```python
from build123d import *

# Parameters (mm, degrees)
F0_R     = 25.4
F0_R_2   = 9.525
F1_DEPTH = 6.35
F2_SIZE  = 5.08


with BuildPart() as f1:
    # F0 (on Front) → F1 (new body)
    with BuildSketch(Plane.XZ):
        with BuildLine():
            Line((109.5375, 0), (1.5875, 0))
            ThreePointArc((1.5875, 0), (1.122532, -1.122532), (0, -1.5875))
            Line((0, -1.5875), (0, -169.8625))
            ThreePointArc((0, -169.8625), (1.122532, -170.327468), (1.5875, -171.45))
            Line((1.5875, -171.45), (109.5375, -171.45))
            ThreePointArc((109.5375, -171.45), (110.002468, -170.327468), (111.125, -169.8625))
            Line((111.125, -169.8625), (111.125, -90.614297))
            ThreePointArc((111.125, -90.614297), (52.3875, -50.8), (111.125, -10.985703))
            Line((111.125, -10.985703), (111.125, -1.5875))
            ThreePointArc((111.125, -1.5875), (110.002468, -1.122532), (109.5375, 0))
        make_face()
        with Locations((77.7875, -142.875)):
            Circle(F0_R, mode=Mode.SUBTRACT)
        with Locations((38.1, -101.6)):
            Circle(F0_R, mode=Mode.SUBTRACT)
        with BuildLine():
            ThreePointArc((0, -1.5875), (-1.122532, 1.122532), (1.5875, 0))
            Line((1.5875, 0), (109.5375, 0))
            ThreePointArc((109.5375, 0), (110.002468, 1.122532), (111.125, 1.5875))
            Line((111.125, 1.5875), (111.125, 14.2875))
            Line((111.125, 14.2875), (-19.05, 14.2875))
            Line((-19.05, 14.2875), (-19.05, -185.7375))
            Line((-19.05, -185.7375), (121.44375, -185.7375))
            Line((121.44375, -185.7375), (121.44375, -129.918501))
            ThreePointArc((121.44375, -129.918501), (135.685573, -89.928697), (174.625, -73.025))
            Line((174.625, -73.025), (174.625, 0))
            Line((174.625, 0), (112.7125, 0))
            ThreePointArc((112.7125, 0), (112.247532, -1.122532), (111.125, -1.5875))
            Line((111.125, -1.5875), (111.125, -10.985703))
            ThreePointArc((111.125, -10.985703), (130.729826, -26.750554), (138.1125, -50.8))
            ThreePointArc((138.1125, -50.8), (130.729826, -74.849446), (111.125, -90.614297))
            Line((111.125, -90.614297), (111.125, -169.8625))
            ThreePointArc((111.125, -169.8625), (112.247532, -170.327468), (112.7125, -171.45))
            ThreePointArc((112.7125, -171.45), (111.125, -173.0375), (109.5375, -171.45))
            Line((109.5375, -171.45), (1.5875, -171.45))
            ThreePointArc((1.5875, -171.45), (-1.122532, -172.572532), (0, -169.8625))
            Line((0, -169.8625), (0, -1.5875))
        make_face()
        with Locations((161.925, -12.7)):
            Circle(F0_R_2, mode=Mode.SUBTRACT)
        with BuildLine():
            Line((234.95, 0), (174.625, 0))
            Line((174.625, 0), (174.625, -73.025))
            ThreePointArc((174.625, -73.025), (212.315461, -88.6369), (227.927361, -126.327361))
            ThreePointArc((227.927361, -126.327361), (227.897074, -128.123951), (227.80625, -129.918501))
            Line((227.80625, -129.918501), (227.80625, -185.7375))
            Line((227.80625, -185.7375), (368.3, -185.7375))
            Line((368.3, -185.7375), (368.3, 14.2875))
            Line((368.3, 14.2875), (236.5375, 14.2875))
            Line((236.5375, 14.2875), (236.5375, 1.5875))
            ThreePointArc((236.5375, 1.5875), (237.660032, 1.122532), (238.125, 0))
            Line((238.125, 0), (347.6625, 0))
            ThreePointArc((347.6625, 0), (349.25, 1.5875), (350.8375, 0))
            ThreePointArc((350.8375, 0), (350.372532, -1.122532), (349.25, -1.5875))
            Line((349.25, -1.5875), (349.25, -169.8625))
            ThreePointArc((349.25, -169.8625), (350.372532, -170.327468), (350.8375, -171.45))
            ThreePointArc((350.8375, -171.45), (349.25, -173.0375), (347.6625, -171.45))
            Line((347.6625, -171.45), (238.125, -171.45))
            ThreePointArc((238.125, -171.45), (235.414968, -172.572532), (236.5375, -169.8625))
            Line((236.5375, -169.8625), (236.5375, -89.944029))
            ThreePointArc((236.5375, -89.944029), (211.1375, -50.8), (236.5375, -11.655971))
            Line((236.5375, -11.655971), (236.5375, -1.5875))
            ThreePointArc((236.5375, -1.5875), (235.414968, -1.122532), (234.95, 0))
        make_face()
        with Locations((187.325, -12.7)):
            Circle(F0_R_2, mode=Mode.SUBTRACT)
        with BuildLine():
            Line((111.125, 14.2875), (111.125, 1.5875))
            ThreePointArc((111.125, 1.5875), (112.247532, 1.122532), (112.7125, 0))
            Line((112.7125, 0), (174.625, 0))
            Line((174.625, 0), (234.95, 0))
            ThreePointArc((234.95, 0), (235.414968, 1.122532), (236.5375, 1.5875))
            Line((236.5375, 1.5875), (236.5375, 14.2875))
            Line((236.5375, 14.2875), (111.125, 14.2875))
        make_face()
        with BuildLine():
            ThreePointArc((238.125, 0), (237.660032, -1.122532), (236.5375, -1.5875))
            Line((236.5375, -1.5875), (236.5375, -11.655971))
            ThreePointArc((236.5375, -11.655971), (277.33139, -14.843914), (296.8625, -50.8))
            ThreePointArc((296.8625, -50.8), (277.33139, -86.756086), (236.5375, -89.944029))
            Line((236.5375, -89.944029), (236.5375, -169.8625))
            ThreePointArc((236.5375, -169.8625), (237.660032, -170.327468), (238.125, -171.45))
            Line((238.125, -171.45), (347.6625, -171.45))
            ThreePointArc((347.6625, -171.45), (348.127468, -170.327468), (349.25, -169.8625))
            Line((349.25, -169.8625), (349.25, -1.5875))
            ThreePointArc((349.25, -1.5875), (348.127468, -1.122532), (347.6625, 0))
            Line((347.6625, 0), (238.125, 0))
        make_face()
        with Locations((271.4625, -142.875)):
            Circle(F0_R, mode=Mode.SUBTRACT)
        with Locations((311.15, -101.6)):
            Circle(F0_R, mode=Mode.SUBTRACT)
    extrude(amount=F1_DEPTH)

    # F2
    f2_edges = [f1.edges().sort_by_distance(p)[0] for p in [
        (174.625, -6.35, 14.2875),
        (298.053125, -6.35, -185.7375),
        (368.3, -6.35, -85.725),
        (51.196875, -6.35, -185.7375),
        (-19.05, -6.35, -85.725),
    ]]
    chamfer(f2_edges, length=F2_SIZE)


solid = f1.part
```
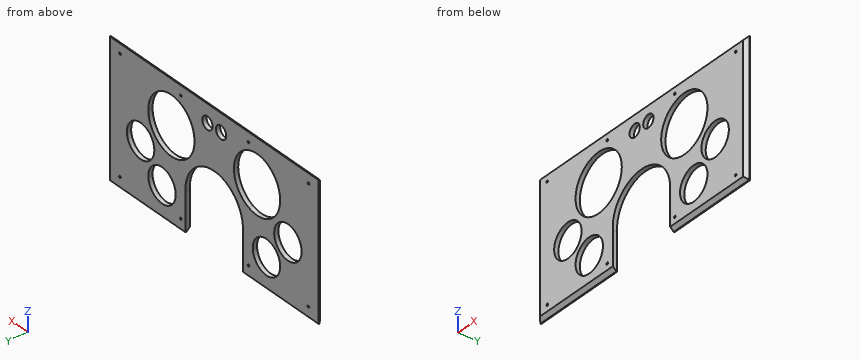
For this review, take the finished solid that the model builds, in its own axes (mm). Round coordinates to 2 decimals unless told otherwise and drop trailing zeros. Write each loop counter-clockwise with the first axis right and the second up, starting at its lowest first coordinate (ties: lowest second). Pieces come first, ordered by that corner, then holes. Notation, with made-up numbers: (11, -15) -> (38, -15) arc R6 ccw to (38, -11) -> close; hole circle Ø7 at (73.5, 45.25). An arc over 180 degrees is marked (long way). Use one line per item in the form item = value.
1) Take a section at D-D, the plane x = 129.5. Write out the cut boundary in (y, z).
Found:
outline = (-6.35, -97.96) -> (0, -97.96) -> (0, -76.57) -> (-6.35, -76.57) -> close; (-6.35, -25.03) -> (0, -25.03) -> (0, 14.29) -> (-1.27, 14.29) -> (-6.35, 9.21) -> close
2) Take a section at B-B, the plane x = 38.1. Write out the cut boundary in (y, z), and give its area (3 significant figures).
Found:
outline = (-6.35, -180.66) -> (-1.27, -185.74) -> (0, -185.74) -> (0, -127) -> (-6.35, -127) -> close; (-6.35, -76.2) -> (0, -76.2) -> (0, 14.29) -> (-1.27, 14.29) -> (-6.35, 9.21) -> close
area = 922 mm2
3) To check wall thickness, follow L1, parallel to Z at x = 262, y = -6; L2, parallel to X at y = -2.75, z = -131; L3, parallel to X at y = -4.5, z = -104.5. State the ranges of each line that lie inside material, in increasing order. Write a range as from..to.
Found:
L1 = -181.01..-166.45, -119.3..-92.91, -8.69..9.56
L2 = -17.57..55.33, 100.24..121.44, 227.81..249.01, 293.92..366.82
L3 = -15.82..12.87, 63.33..126, 223.25..285.92, 336.38..365.07
4) Take a section at A-A, the plane z = -101.6. Write out the cut boundary in (x, y).
Found:
outline = (-19.05, -1.27) -> (-13.97, -6.35) -> (12.7, -6.35) -> (12.7, 0) -> (-19.05, 0) -> close; (63.5, -6.35) -> (127.41, -6.35) -> (127.41, 0) -> (63.5, 0) -> close; (221.84, -6.35) -> (285.75, -6.35) -> (285.75, 0) -> (221.84, 0) -> close; (336.55, -6.35) -> (363.22, -6.35) -> (368.3, -1.27) -> (368.3, 0) -> (336.55, 0) -> close
5) Clearance check with flat-ended pins moving along their axes: pin 1 (11.5 mm diameter, centred on x = 161.925, z = -12.7, fed in from -Y); pin 2 (22 mm diameter, centred on x = 187.325, z = -12.7, fed in from -Y); pin 3 (2 mm diameter, centred on x = 251, y = -3, fed in from +Z); pin 4 (3 mm diameter, centred on y = -3.5, z = -33, fed in from -X). State where each tip first meets the part, or that it passes through.
Found:
pin_1 = through
pin_2 = -6.35
pin_3 = 13.56
pin_4 = -18.32
6) Take a section at C-C, the plane y = -3.25. Count the separate pieces of the cut face and the enclosed holes in it, and give its area (3 significant figures).
Found:
separate_pieces = 1
enclosed_holes = 16
area = 44,300 mm2
